Geometry: final body of the model. Coordinates: model frame, mm. Face numbers are marked on the shaded views. A direction names the side the tool comes from. Give positions to 0.01 mm unless a question says otherwise; leave off trailing zeros. Order: outer loops, then holes, each group sorted by start corner. A loop starts at its lowest first (then second) coordinate and runs counter-clockwise, first axis right, second up. Notation, with made-up numbers: (73, -35.5) -> (121, -35.5) arc R21 cw to (121, -0.5) -> close; hole circle Ø10 at (12, 29). An arc over 180 degrees is marked (long way). One line per question, with ' | ' between items.
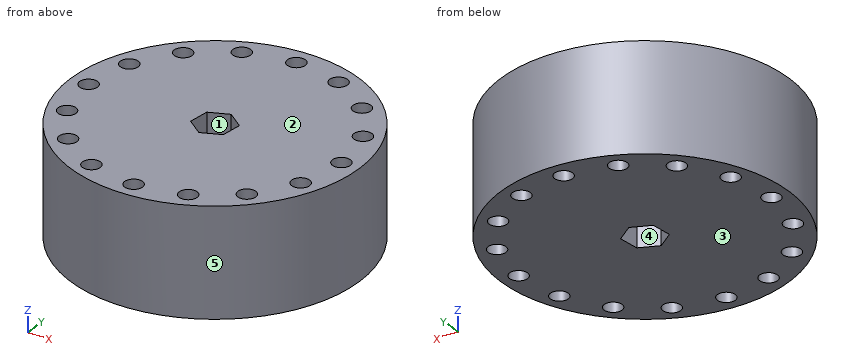
from build123d import *

# Parameters (mm, degrees)
SKETCH1_R           = 50.8
BOSS_EXTRUDE1_DEPTH = 38.1
SKETCH2_R           = 3.175
CUT_EXTRUDE1_DEPTH  = 39.1


with BuildPart() as part:
    # Sketch1 → Boss-Extrude1 (new body)
    with BuildSketch(Plane.XY):
        Circle(SKETCH1_R)
        Polygon((5.789348381, -4.499642059), (6.791478521, 2.76390174), (1.00213014, 7.263543799), (-5.789348381, 4.499642059), (-6.791478521, -2.76390174), (-1.00213014, -7.263543799), align=None, mode=Mode.SUBTRACT)
    extrude(amount=BOSS_EXTRUDE1_DEPTH)

    # Sketch2 → Cut-Extrude1 (cut, through all)
    with BuildSketch(Plane.XY.offset(38.1)):
        with Locations((0, 44.377138181)):
            Circle(SKETCH2_R)
        with Locations((16.982395558, 40.999129677)):
            Circle(SKETCH2_R)
        with Locations((31.379375337, 31.379375337)):
            Circle(SKETCH2_R)
        with Locations((40.999129677, 16.982395558)):
            Circle(SKETCH2_R)
        with Locations((44.377138181, 0)):
            Circle(SKETCH2_R)
        with Locations((40.999129677, -16.982395558)):
            Circle(SKETCH2_R)
        with Locations((31.379375337, -31.379375337)):
            Circle(SKETCH2_R)
        with Locations((16.982395558, -40.999129677)):
            Circle(SKETCH2_R)
        with Locations((0, -44.377138181)):
            Circle(SKETCH2_R)
        with Locations((-16.982395558, -40.999129677)):
            Circle(SKETCH2_R)
        with Locations((-31.379375337, -31.379375337)):
            Circle(SKETCH2_R)
        with Locations((-40.999129677, -16.982395558)):
            Circle(SKETCH2_R)
        with Locations((-44.377138181, 0)):
            Circle(SKETCH2_R)
        with Locations((-40.999129677, 16.982395558)):
            Circle(SKETCH2_R)
        with Locations((-31.379375337, 31.379375337)):
            Circle(SKETCH2_R)
        with Locations((-16.982395558, 40.999129677)):
            Circle(SKETCH2_R)
    extrude(amount=-CUT_EXTRUDE1_DEPTH, mode=Mode.SUBTRACT)


solid = part.part
1) Section A-A on y = 0. Return loops of the section in (x, z).
Check result:
outline: (-50.8, 0) -> (-47.55, 0) -> (-47.55, 38.1) -> (-50.8, 38.1) -> close; (-41.2, 0) -> (-6.41, 0) -> (-6.41, 38.1) -> (-41.2, 38.1) -> close; (6.41, 0) -> (41.2, 0) -> (41.2, 38.1) -> (6.41, 38.1) -> close; (47.55, 0) -> (50.8, 0) -> (50.8, 38.1) -> (47.55, 38.1) -> close
2) Section B-B on z = 33. Count the separate pieces of the cut face and the enclosed holes in it, plus the area to 3 significant figures.
Check result:
separate pieces: 1 | enclosed holes: 17 | area: 7,460 mm^2
3) Contact query for flat-ended pins moving along their axis: pin 1 Ø8 at (y, z) = (-33.5, 17.5) entering from -X; pin 2 Ø12 at (x, y) = (-37.5, 35) entering from +Z; pin 3 Ø4 at (x, y) = (41, 16.98) entering from +Z; pin 4 Ø8 at (x, z) = (29, 32.5) entering from -Y. Output: stop coordinate, or through.
Check result:
pin 1: stops at x = -41.36 | pin 2: stops at z = 38.1 | pin 3: passes through | pin 4: stops at y = -44.22
4) Material intervals for probe 1 along Y at (x, z) = (-43.5, 13.5); probe 2 along X at (y, z) = (-42, 27); probe 3 along Y at (x, z) = (0, 12), sorted ascending. Write a range as from..to.
Check result:
probe 1: y = -26.24..-18.94, -15.03..-3.05, 3.05..15.03, 18.94..26.24 | probe 2: x = -28.58..-20, -13.97..-2.1, 2.1..13.97, 20..28.58 | probe 3: y = -50.8..-47.55, -41.2..-6.86, 6.86..41.2, 47.55..50.8
5) Pull-direction query (Y, two-part tool) for the marked faces 3, 4 and 5; classes: +Y half, -Y half, draft (parallel to the pull), parting line (faces both ways), or undercut.
Check result:
face 3: draft | face 4: undercut | face 5: parting line
6) Set-up query: the marked faces 1 and 2. Return all of +Z, -Z, +X, -X, +Y, -Y with unobstructed straight access to the full face (end or side cutting, diameter ignored); none if empty.
Check result:
face 1: +Z, -Z | face 2: +Z, +X, -X, +Y, -Y
